Geometry check sheet. Reference: the model listing, model coordinates, mm. A direction names the side the tool comes from. Round coordinates to 2 decimals unless told otherwise and drop trailing zeros. Order: outer loops, then holes, each group sorted by start corner. A loop starts at its lowest first (then second) coordinate and runs counter-clockwise, first axis right, second up. Notation, with made-up numbers: M 73,-19.5 L 101,-19.5 A32 ccw 101,8.5 Z; hole C 65,76 d8. An arc over 180 degrees is marked long. Answer as a JSON object with one key per item and string values. Group by question number.
Autodesk Inventor part; units mm, degrees
ref_plane "YZ Plane" through (0, 0, 0) normal (1, 0, 0) x (0, 1, 0)
ref_plane "XZ Plane" through (0, 0, 0) normal (0, 1, 0) x (-1, 0, 0)
ref_plane "XY Plane" through (0, 0, 0) normal (0, 0, 1) x (1, 0, 0)
sketch "Sketch1" plane through (0, 0, 0) normal (1, 0, 0) x (0, 1, 0)
  line L0 (31.75, 82.55) -> (-31.75, 82.55)
  line L1 (-31.75, 82.55) -> (-31.75, -82.55)
  line L2 (-31.75, -82.55) -> (31.75, -82.55)
  line L3 (31.75, -82.55) -> (31.75, 82.55)
  point P0 (0, 0)
  point P1 (31.75, 0)
  point P2 (0, 82.55)
  dimension "d0" = 165.1
  dimension "d1" = 63.5
extrude "Extrusion1" add sketch "Sketch1" along normal blind 9.525
sketch "Sketch3" plane through (9.525, 0, 0) normal (1, 0, 0) x (0, 0, -1)
  line L0 (72.898, -22.098) -> (-72.898, -22.098)
  line L1 (-72.898, -22.098) -> (-72.898, 22.098)
  line L2 (-72.898, 22.098) -> (72.898, 22.098)
  line L3 (72.898, 22.098) -> (72.898, -22.098)
  line L4 (72.898, -22.098) -> (-72.898, 22.098) construction
  line L5 (-72.898, -22.098) -> (72.898, 22.098) construction
  line L6 (79.375, -28.575) -> (-79.375, -28.575)
  line L7 (-79.375, -28.575) -> (-79.375, 28.575)
  line L8 (-79.375, 28.575) -> (79.375, 28.575)
  line L9 (79.375, 28.575) -> (79.375, -28.575)
  line L10 (79.375, -28.575) -> (-79.375, 28.575) construction
  line L11 (-79.375, -28.575) -> (79.375, 28.575) construction
  point P0 (0, 0)
  point P1 (0, 0)
  point P2 (0, 0)
  dimension "d16" = 145.796
  dimension "d17" = 44.196
  dimension "d18" = 6.477
  dimension "d19" = 6.477
extrude "Extrusion3" cut sketch "Sketch3" against normal blind 3.175
fillet "Fillet1" radius 3.175 8 edges at (7.9375, -28.575, 79.375) (7.9375, 28.575, 79.375) (7.9375, 28.575, -79.375) (7.9375, -28.575, -79.375) (7.9375, -22.098, 72.898) (7.9375, 22.098, 72.898) (7.9375, 22.098, -72.898) (7.9375, -22.098, -72.898)
equation "\"d0\" = tubeWidth + 2 * plateOverhang"
equation "\"d1\" = tubeHeight + 2 * plateOverhang"
equation "\"d2\" = blankCapThickness"
equation "\"d16\" = -2 * tubeWallThickness + tubeWidth - 2 * tubePlateClearance"
equation "\"d17\" = -2 * tubeWallThickness + tubeHeight - 2 * tubePlateClearance"
equation "\"d18\" = tubeWallThickness + tubePlateClearance + moatWidth"
equation "\"d19\" = tubeWallThickness + tubePlateClearance + moatWidth"
equation "\"d12\" = moatDepth"
equation "\"tubeHeight\" = 50.8"
equation "\"tubeWidth\" = 152.4"
equation "\"tubeLength\" = 304.8"
equation "\"tubeWallThickness\" = 3.175"
equation "\"plateOverhang\" = 6.35"
equation "\"moatWidth\" = 3.175"
equation "\"tubePlateClearance\" = 0.127"
equation "\"moatDepth\" = 3.175"
equation "\"blankCapThickness\" = 9.525"
equation "\"fiberClearance\" = 0"
equation "\"oRingID\" = 22.2504"
equation "\"fiberDiameter\" = 1"
equation "\"sensorHolderThickness\" = 12.7"
equation "\"oRingGrooveWidth\" = 2.54"
equation "\"longHoleSpacing\" = 30.48"
equation "\"sensorHolderDiameter\" = 50.8"
equation "\"shortHoleSpacing\" = 21.59"
equation "\"glassTubeClearance\" = 0.19844"
equation "\"glassTubeDiameter\" = 12.7"
equation "\"sensorCapThickness\" = 12.7"
equation "\"oRingGrooveDepth\" = 1.2446"
equation "\"glassTubeID\" = 7.874"
equation "\"glassTubeLength\" = 279.4"
equation "\"sensorBoardHoleSpacing\" = 19"
properties part number "plateEnd" material "Aluminum 6061"
1) Sectioned sample at A-A (z = -11). Record the boundary of the cut face in (x, y) (3 decimals), then the cut area to 3 significant figures.
2) Release check for a two-part mould opening along Z. For faces 1 (the flat face through (9.525, -31, 25)), 2 (the flat face through (5, 0, -82.55)), 3 (the flat face through (6.35, -23, 6)) record: +Z half, -Z half, draft (parallel to the pull), parting line (faces both ways), or undercut.
3) Thickness scan on line 1 along Z through (x, y) = (8.25, 3.5) (3 decimals); line 2 along Y through (x, z) = (9.25, -2) (3 decimals); line 3 along Z through (x, y) = (8.5, -25) (3 decimals). Record the ranges inside material, lowest first. Write a range as [from, to].
4) Set-up check for faces 4 (the flat face through (0, 0, 1)), 5 (the flat face through (8, 0, 79.375)): record each of +Z, -Z, +X, -X, +Y, -Y from which the full face is reachable in a straight line by a thin tool's end or side.
5) Sectioned sample at B-B (y = 8). Record the boundary of the cut face in (x, z) (3 decimals), then the cut area to 3 significant figures.
Final values:
{
 "1": {"outline": "M 0,-31.75 L 9.525,-31.75 L 9.525,-28.575 L 6.35,-28.575 L 6.35,-22.098 L 9.525,-22.098 L 9.525,22.098 L 6.35,22.098 L 6.35,28.575 L 9.525,28.575 L 9.525,31.75 L 0,31.75 Z", "area": "564 mm^2"},
 "2": {"face 1": "draft", "face 2": "-Z half", "face 3": "undercut"},
 "3": {"line 1": "z = [-82.55, -79.375], [-72.898, 72.898], [79.375, 82.55]", "line 2": "y = [-31.75, -28.575], [-22.098, 22.098], [28.575, 31.75]", "line 3": "z = [-82.55, -79.375], [79.375, 82.55]"},
 "4": {"face 4": "+Z, -Z, -X, +Y, -Y", "face 5": "+X"},
 "5": {"outline": "M 0,-82.55 L 9.525,-82.55 L 9.525,-79.375 L 6.35,-79.375 L 6.35,-72.898 L 9.525,-72.898 L 9.525,72.898 L 6.35,72.898 L 6.35,79.375 L 9.525,79.375 L 9.525,82.55 L 0,82.55 Z", "area": "1,530 mm^2"}
}
